The listing builds one solid part. Answer for the finished solid, in the listing's coordinates (mm). Round coordinates to 2 decimals unless told otherwise and drop trailing zeros. Return JSON: item names as keys, results as strings. Group by question number.
from build123d import *

# Parameters (mm, degrees)
F0_R     = 1.5
F0_R_2   = 1.875
F1_DEPTH = 1.8


with BuildPart() as f1:
    # F0 (on Top) → F1 (new body)
    with BuildSketch(Plane.XY):
        with BuildLine():
            Line((-98.341699, -18.824226), (-4.341699, -18.824226))
            ThreePointArc((-4.341699, -18.824226), (-2.220379, -17.945546), (-1.341699, -15.824226))
            Line((-1.341699, -15.824226), (-1.341699, 84.175774))
            ThreePointArc((-1.341699, 84.175774), (-2.220379, 86.297094), (-4.341699, 87.175774))
            Line((-4.341699, 87.175774), (-98.341699, 87.175774))
            ThreePointArc((-98.341699, 87.175774), (-100.46302, 86.297094), (-101.341699, 84.175774))
            Line((-101.341699, 84.175774), (-101.341699, -15.824226))
            ThreePointArc((-101.341699, -15.824226), (-100.46302, -17.945546), (-98.341699, -18.824226))
        make_face()
        with Locations((-94.341699, -11.824226)):
            Circle(F0_R, mode=Mode.SUBTRACT)
        with Locations((-83.92407, 28.841723)):
            Circle(F0_R, mode=Mode.SUBTRACT)
        with Locations((-63.92407, 28.841723)):
            Circle(F0_R, mode=Mode.SUBTRACT)
        with Locations((-91.388723, 60.224189)):
            Circle(F0_R, mode=Mode.SUBTRACT)
        with Locations((-94.341699, 80.175774)):
            Circle(F0_R, mode=Mode.SUBTRACT)
        with Locations((-38.428727, -8.937866)):
            Circle(F0_R_2, mode=Mode.SUBTRACT)
        with Locations((-8.341699, -11.824226)):
            Circle(F0_R, mode=Mode.SUBTRACT)
        with Locations((-11.03972, 21.549158)):
            Circle(F0_R_2, mode=Mode.SUBTRACT)
        with Locations((-45.174403, 60.224189)):
            Circle(F0_R, mode=Mode.SUBTRACT)
        with Locations((-31.175356, 40.833933)):
            Circle(F0_R, mode=Mode.SUBTRACT)
        with Locations((-8.341699, 80.175774)):
            Circle(F0_R, mode=Mode.SUBTRACT)
    extrude(amount=F1_DEPTH)


solid = f1.part
(1) A flat-ended cylindrical pin translates along its axis: pin 1 (6 mm diameter, centred on x = -29.5, y = 66, fed in from -Z). Find the tip coordinate at first contact, or state that the pin passes through.
(2) Determine the mould class of faces 1 (the cylindrical face through (-100.44, 86.32, 0.89)), 2 (the cylindrical face through (-83.12, 30.11, 0.89)), 3 (the flat face through (-52, 35, 0)) for opening direction X: +X half, -X half, draft (parallel to the pull), parting line (faces both ways), or undercut.
(3) Consider line 1 (X direction, y = -9, z = 0.8); line 2 (Y direction, x = -92, z = 0.35); line 3 (Y direction, x = -7, z = 0.5). Determine where each line is inside the solid, lowest interval first.
Check sheet entries:
{
 "1": {"pin 1": "stops at z = 0"},
 "2": {"face 1": "-X half", "face 2": "undercut", "face 3": "draft"},
 "3": {"line 1": "x = -101.34 to -40.3, -36.55 to -1.34", "line 2": "y = -18.82 to 58.85, 61.59 to 87.18", "line 3": "y = -18.82 to -12.49, -11.15 to 79.51, 80.85 to 87.18"}
}
